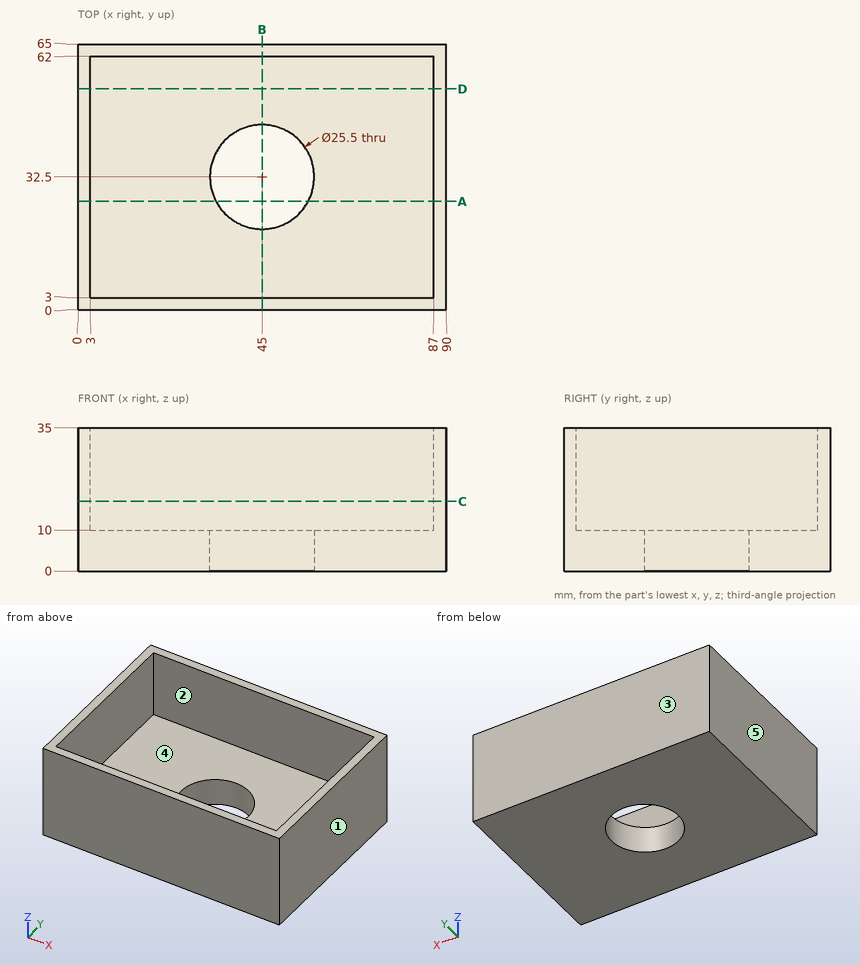
The drawing under review shows one solid part. Ordinate dimensions are in mm from its lowest x, y, z. A direction names the side the tool comes from. Round coordinates to 2 decimals unless told otherwise and drop trailing zeros. Write each loop counter-clockwise with the first axis right and the second up, starting at its lowest first coordinate (ties: lowest second). Pieces come first, ordered by that corner, then holes. Notation, with made-up numbers: (11.5, -12) -> (62.5, -12) arc R22 cw to (62.5, 4) -> close; hole circle Ø1 at (18.5, 50.5). An arc over 180 degrees is marked (long way). Put each result on its own line as item: value.
Q1. To check wall thickness, follow L1, parallel to Y at x = 56, z = 16.5; L2, parallel to X at y = 7.5, z = 24.5; L3, parallel to X at y = 32, z = 6. State the ranges of each line that lie inside material, in increasing order. Write a range as [from, to].
Determined:
L1: y = [0, 3], [62, 65]
L2: x = [0, 3], [87, 90]
L3: x = [0, 32.26], [57.74, 90]
Q2. Consider section D-D on y = 54. State the section outline as (x, z) points.
Determined:
outline: (0, 0) -> (90, 0) -> (90, 35) -> (87, 35) -> (87, 10) -> (3, 10) -> (3, 35) -> (0, 35) -> close
Q3. Consider section A-A on y = 26.5. State the section outline as (x, z) points, and give its area (3 significant figures).
Determined:
outline: (0, 0) -> (33.75, 0) -> (33.75, 10) -> (3, 10) -> (3, 35) -> (0, 35) -> close; (56.25, 0) -> (90, 0) -> (90, 35) -> (87, 35) -> (87, 10) -> (56.25, 10) -> close
area: 825 mm^2
Q4. Consider section B-B on x = 45. State the section outline as (y, z) points, and give its area (3 significant figures).
Determined:
outline: (0, 0) -> (19.75, 0) -> (19.75, 10) -> (3, 10) -> (3, 35) -> (0, 35) -> close; (45.25, 0) -> (65, 0) -> (65, 35) -> (62, 35) -> (62, 10) -> (45.25, 10) -> close
area: 545 mm^2
Q5. Clearance check with flat-ended pins moving along their axes: pin 1 Ø23 at (x, y) = (45, 32.5) entering from -Z; pin 2 Ø17.5 at (x, y) = (41.5, 45) entering from +Z. State where each tip first meets the part, or that it passes through.
Determined:
pin 1: passes through
pin 2: stops at z = 10
Q6. The part is to be moulded in two halves that separate along X. For the marked faces 3, 4 and 5, say which applies: released by +X, released by -X, zero draft, split by the parting line, or undercut.
Determined:
face 3: zero draft
face 4: undercut
face 5: released by -X
Q7. Consider section C-C on z = 17. State the section outline as (x, y) points, and give its area (3 significant figures).
Determined:
outline: (0, 0) -> (90, 0) -> (90, 65) -> (0, 65) -> close; hole (3, 3) -> (87, 3) -> (87, 62) -> (3, 62) -> close
area: 894 mm^2
Q8. Machinability: for the marked faces 1 and 2, which of the approach directions +Z, -Z, +X, -X, +Y, -Y give a long, thin tool a straight path to every point of the face, cutting with its end or side? Answer none if there is none.
Determined:
face 1: +Z, -Z, +X, +Y, -Y
face 2: +Z
